from build123d import *

# Parameters (mm, degrees)
SKETCH064_W            = 93
SKETCH064_H            = 73
PAD021_DEPTH           = 3
FILLET016_R            = 4
SKETCH065_R            = 1.65
POCKET045_DEPTH        = 3.001
SKETCH069_W            = 6
SKETCH069_H            = 30
PAD023_DEPTH           = 3
CHAMFER016_SIZE        = 1
POCKET050_DEPTH        = 3.001
LINEARPATTERN001_COUNT = 4
LINEARPATTERN001_PITCH = 10


with BuildPart() as part:
    # Sketch064 (on Face1 of CopyMirrored003) → Pad021 (new body)
    with BuildSketch(Plane(origin=(0, 0, 0), x_dir=(1, 0, 0), z_dir=(0, 0, -1))):
        Rectangle(SKETCH064_W, SKETCH064_H)
    extrude(amount=PAD021_DEPTH)

    # Fillet016
    fillet016_edges = [part.edges().sort_by_distance(p)[0] for p in [
        (-46.5, 36.5, -1.5),
        (-46.5, -36.5, -1.5),
        (46.5, -36.5, -1.5),
        (46.5, 36.5, -1.5),
    ]]
    fillet(fillet016_edges, radius=FILLET016_R)

    # Sketch065 (on Face5 of Fillet016) → Pocket045 (cut, through all)
    with BuildSketch(Plane(origin=(0, 0, -3), x_dir=(1, 0, 0), z_dir=(0, 0, -1))):
        with Locations((-40, 30)):
            Circle(SKETCH065_R)
        with Locations((-40, -30)):
            Circle(SKETCH065_R)
        with Locations((40, 30)):
            Circle(SKETCH065_R)
        with Locations((40, -30)):
            Circle(SKETCH065_R)
    extrude(amount=-POCKET045_DEPTH, mode=Mode.SUBTRACT)

    # Sketch069 (on Face5 of Pocket045) → Pad023 (join)
    with BuildSketch(Plane(origin=(0, 0, -3), x_dir=(1, 0, 0), z_dir=(0, 0, -1))):
        with Locations((-49.5, 0)):
            Rectangle(SKETCH069_W, SKETCH069_H)
    extrude(amount=-PAD023_DEPTH)

    # Chamfer016
    chamfer016_edges = [part.edges().sort_by_distance(p)[0] for p in [
        (-52.5, 15, -1.5),
        (-52.5, -15, -1.5),
        (-46.5, -15, -1.5),
        (-46.5, 15, -1.5),
    ]]
    chamfer(chamfer016_edges, length=CHAMFER016_SIZE)

    # Sketch073 (on Face5 of Chamfer016) → Pocket050 (cut, through all)
    with BuildSketch(Plane(origin=(0, 0, -3), x_dir=(1, 0, 0), z_dir=(0, 0, -1))):
        with BuildLine():
            ThreePointArc((-32, 20), (-34, 22), (-36, 20))
            Line((-36, 20), (-36, -20))
            ThreePointArc((-36, -20), (-34, -22), (-32, -20))
            Line((-32, 20), (-32, -20))
        make_face()
    pocket050 = extrude(amount=-POCKET050_DEPTH, mode=Mode.SUBTRACT)

    # LinearPattern001: Pocket050 ×4
    with Locations(*[(i * LINEARPATTERN001_PITCH, 0, 0) for i in range(1, LINEARPATTERN001_COUNT)]):
        add(pocket050, mode=Mode.SUBTRACT)


solid = part.part
Can you work these out from the model? Positions are in its coordinate system, mm. A direction names the side the tool comes from. Coordinates: 2 decimals unless noted, no trailing zeros. Order: outer loops, then holes, each group sorted by start corner. A loop starts at its lowest first (then second) coordinate and runs counter-clockwise, first axis right, second up. Notation, with made-up numbers: (-11.5, 70.25) - (-0.5, 70.25) arc R13 ccw to (-0.5, 91.25) - close; hole circle Ø3 at (46.5, 66.5). An arc over 180 degrees is marked (long way). Answer as a JSON object with one key per item and string values. Group by question number.
Q1. Imagine slicing it at C-C (y = 30). Please give me the cut outline in (x, z), and give its area (3 significant figures).
Q2. We'd pull the mould along X, two halves only. Please class faces 4 (the face through (-12, 0, -2)), 5 (the face through (46.5, 0, -1)), 6 (the face through (-52.5, 0, -2)), 7 (the face through (7, -1, 0)): +X half, -X half, draft (parallel to the pull), parting line (faces both ways), or undercut.
Q3. Imagine slicing it at B-B (x = -4). Please give me the cut outline in (y, z).
Q4. Imagine slicing it at A-A (y = -6). Please give me the cut outline in (x, z), and give its area (3 significant figures).
Q5. Imagine slicing it at D-D (x = 40). Please give me the cut outline in (y, z), and give its area (3 significant figures).
Q6. On a 3-axis mill with a long thin cutter (end or side, diameter ignored), from which of +Z, -Z, +X, -X, +Y, -Y can I reach the whole of each face in a straight line? I mean faces 1 (the face through (-16, 0, -2)), 2 (the face through (45.297, 35.359, -1.521)), 3 (the face through (-50, 15, -2)). Say none if no direction works.
Q7. Will these pins go through, and if not, where does the flat tip stop? P1, Ø1.5, axis at x = -50, z = -1, coming from the -Y side; P2, Ø0.9, axis at y = 27.5, z = -1.5, coming from the -X side.
Q8. I need wall thicknesses on line 1 (X direction, y = -30, z = -1.2); line 2 (X direction, y = -17, z = -0.6); line 3 (Y direction, x = -40, z = -1.05). Which ranges of each line are inside material? Lowest first, please. Write a range as from..to.
Determined:
{
 "1": {"outline": "(-46.5, -3) - (-41.65, -3) - (-41.65, 0) - (-46.5, 0) - close; (-38.35, -3) - (38.35, -3) - (38.35, 0) - (-38.35, 0) - close; (41.65, -3) - (46.5, -3) - (46.5, 0) - (41.65, 0) - close", "area": "259 mm2"},
 "2": {"face 4": "undercut", "face 5": "+X half", "face 6": "-X half", "face 7": "draft"},
 "3": {"outline": "(-36.5, -3) - (-22, -3) - (-22, 0) - (-36.5, 0) - close; (22, -3) - (36.5, -3) - (36.5, 0) - (22, 0) - close"},
 "4": {"outline": "(-52.5, -3) - (-36, -3) - (-36, 0) - (-52.5, 0) - close; (-32, -3) - (-26, -3) - (-26, 0) - (-32, 0) - close; (-22, -3) - (-16, -3) - (-16, 0) - (-22, 0) - close; (-12, -3) - (-6, -3) - (-6, 0) - (-12, 0) - close; (-2, -3) - (46.5, -3) - (46.5, 0) - (-2, 0) - close", "area": "249 mm2"},
 "5": {"outline": "(-36.5, -3) - (-31.65, -3) - (-31.65, 0) - (-36.5, 0) - close; (-28.35, -3) - (28.35, -3) - (28.35, 0) - (-28.35, 0) - close; (31.65, -3) - (36.5, -3) - (36.5, 0) - (31.65, 0) - close", "area": "199 mm2"},
 "6": {"face 1": "+Z, -Z", "face 2": "+Z, -Z, +X, +Y", "face 3": "+Z, -Z, -X, +Y"},
 "7": {"P1": "stops at y = -15", "P2": "stops at x = -46.5"},
 "8": {"line 1": "x = -46.5..-41.65, -38.35..38.35, 41.65..46.5", "line 2": "x = -46.5..-36, -32..-26, -22..-16, -12..-6, -2..46.5", "line 3": "y = -36.5..-31.65, -28.35..28.35, 31.65..36.5"}
}
